The listing builds one solid part. Answer for the finished solid, in the listing's coordinates (mm). Round coordinates to 2 decimals unless told otherwise and drop trailing zeros. Write each loop counter-clockwise with the first axis right and the second up, starting at its lowest first coordinate (ties: lowest second). Pieces come first, ordered by that corner, then holes.
(1) Each of these flat-tipped pins is pushed along its axis until it touches: pin 1 Ø2 at (y, z) = (5, -11) entering from -X; pin 2 Ø5 at (x, z) = (7, 9.5) entering from -Y; pin 3 Ø3 at (y, z) = (-7, -2.5) entering from -X; pin 4 Ø4 at (y, z) = (5.5, -4.5) entering from -X. Where does it stop, or does it pass through?
(2) A cutting plane is placed at A-A, the plane y = -5. Give the vertices of the cut face in (x, z).
(3) Find the intervals of material crossed by probe 1 along X at (y, z) = (-3, 0); probe 2 along X at (y, z) = (5.75, -9); probe 3 along Z at (x, y) = (5, -5), in increasing order.
(4) The mould has two halves that part along X. Classify faces 1 (the face through (-11.712, -8.273, -20.172)), 2 (the face through (3.755, -0.123, 11.923)), 3 (the face through (23.33, -8.27, -0.06)): +X half, -X half, draft (parallel to the pull), parting line (faces both ways), or undercut.
from build123d import *

# Parameters (mm, degrees)
SKETCH3_R               = 12.5
BOSS_EXTRUDE1_DEPTH     = 8.75
SKETCH4_OUTSIDE_W       = 75.076
SKETCH4_OUTSIDE_H       = 68.114
SKETCH4_OUTSIDE_R       = 22.5
CUT_EXTRUDE1_DEPTH      = 2
CUT_EXTRUDE1_DRAFT      = -60
MIRROR1_COPY_1_SKETCH_W = 75.076
MIRROR1_COPY_1_SKETCH_H = 68.114
MIRROR1_COPY_1_SKETCH_R = 22.5
MIRROR1_COPY_1_DEPTH    = 2
MIRROR1_COPY_1_DRAFT    = -60


with BuildPart() as part:
    # Sketch3 → Boss-Extrude1 (new, symmetric)
    with BuildSketch(Plane(origin=(0, 0, 0), x_dir=(1, 0, 0), z_dir=(0, 1, 0))):
        Polygon((25.980762114, 0), (12.990381057, 22.5), (-12.990381057, 22.5), (-25.980762114, 0), (-12.990381057, -22.5), (12.990381057, -22.5), align=None)
        with Locations(Location((0, 0, 0), (0, 0, 270))):
            Circle(SKETCH3_R, mode=Mode.SUBTRACT)
    extrude(amount=BOSS_EXTRUDE1_DEPTH, both=True)


with BuildPart() as cut_extrude1_tool:
    # Sketch4 outside → Cut-Extrude1 (with draft: the straight prism first)
    with BuildSketch(Plane.XZ.offset(8.75)):
        Rectangle(SKETCH4_OUTSIDE_W, SKETCH4_OUTSIDE_H)
        Circle(SKETCH4_OUTSIDE_R, mode=Mode.SUBTRACT)
    extrude(amount=-CUT_EXTRUDE1_DEPTH)
    # Cut-Extrude1: the draft: its side faces are tilted about the plane it starts from
    cut_extrude1_sides = [cut_extrude1_tool.faces().sort_by_distance(p)[0] for p in [
        (0, -7.75, -34.057),
        (37.538, -7.75, 0),
        (0, -7.75, 34.057),
        (-37.538, -7.75, 0),
        (-22.5, -7.75, 0),
    ]]
    draft(cut_extrude1_sides, Plane.XZ.offset(8.75), CUT_EXTRUDE1_DRAFT)


with BuildPart() as part_1:
    add(part.part)

    # Cut-Extrude1: cut by cut_extrude1_tool
    add(cut_extrude1_tool.part, mode=Mode.SUBTRACT)


with BuildPart() as mirror1_copy_1_tool:
    # Mirror1 copy 1 sketch → Mirror1 copy 1 (with draft: the straight prism first)
    with BuildSketch(Plane(origin=(0, 8.75, 0), x_dir=(1, 0, 0), z_dir=(0, 1, 0))):
        Rectangle(MIRROR1_COPY_1_SKETCH_W, MIRROR1_COPY_1_SKETCH_H)
        Circle(MIRROR1_COPY_1_SKETCH_R, mode=Mode.SUBTRACT)
    extrude(amount=-MIRROR1_COPY_1_DEPTH)
    # Mirror1 copy 1: the draft: its side faces are tilted about the plane it starts from
    mirror1_copy_1_sides = [mirror1_copy_1_tool.faces().sort_by_distance(p)[0] for p in [
        (0, 7.75, -34.057),
        (37.538, 7.75, 0),
        (0, 7.75, 34.057),
        (-37.538, 7.75, 0),
        (-22.5, 7.75, 0),
    ]]
    draft(mirror1_copy_1_sides, Plane(origin=(0, 8.75, 0), x_dir=(1, 0, 0), z_dir=(0, 1, 0)), MIRROR1_COPY_1_DRAFT)


with BuildPart() as part_2:
    add(part_1.part)

    # Mirror1 copy 1: cut by mirror1_copy_1_tool
    add(mirror1_copy_1_tool.part, mode=Mode.SUBTRACT)


solid = part_2.part
Solutions:
1. pin 1: stops at x = -20.21
1. pin 2: stops at y = -8.75
1. pin 3: stops at x = -25.4
1. pin 4: stops at x = -24.54
2. outline: (-25.98, 0) - (-12.99, -22.5) - (12.99, -22.5) - (25.98, 0) - (12.99, 22.5) - (-12.99, 22.5) - close; hole circle Ø25 at (0, 0)
3. probe 1: x = -25.98 to -12.5, 12.5 to 25.98
3. probe 2: x = -20.78 to -8.67, 8.67 to 20.78
3. probe 3: z = -22.5 to -11.46, 11.46 to 22.5
4. face 1: -X half
4. face 2: undercut
4. face 3: +X half
